from build123d import *

# Parameters (mm, degrees)
F0_W      = 25.4
F0_H      = 25.4
F1_DEPTH  = 25.4
F2_R      = 2.53667
F3_DEPTH  = 5.08
F4_R      = 2.54
F5_DEPTH  = 5.08
F6_R      = 2.54
F7_DEPTH  = 5.08
F8_R      = 2.543532
F9_DEPTH  = 5.08
F10_R     = 2.54
F11_DEPTH = 5.08
F12_R     = 2.54
F13_DEPTH = 5.08
F14_R     = 2.54
F15_DEPTH = 5.08
F16_R     = 2.54
F18_DEPTH = 5.08
F17_R     = 2.54
F19_DEPTH = 5.08
F20_R     = 2.54
F24_DEPTH = 5.08
F23_R     = 2.54
F25_DEPTH = 5.08
F22_R     = 2.54
F26_DEPTH = 5.08
F21_R     = 2.54
F27_DEPTH = 5.08
F28_R     = 2.54
F29_DEPTH = 5.08
F31_R     = 2.54
F32_DEPTH = 5.08
F30_R     = 2.54
F33_DEPTH = 5.08
F34_R     = 2.54
F35_DEPTH = 5.08
F36_R     = 2.54
F37_DEPTH = 5.08
F38_R     = 2.54
F39_DEPTH = 5.08
F40_R     = 2.54
F41_DEPTH = 5.08
F42_R     = 2.54
F43_DEPTH = 5.08


with BuildPart() as f1:
    # F0 (on Top) → F1 (new body)
    with BuildSketch(Plane.XY):
        with Locations((-141.267316, -86.385182)):
            Rectangle(F0_W, F0_H)
    extrude(amount=F1_DEPTH)

    # F2 (on face) → F3 (cut)
    with BuildSketch(Plane(origin=(-153.967316, 0, 0), x_dir=(0, -1, 0), z_dir=(-1, 0, 0))):
        with Locations((86.594619, 12.688329)):
            Circle(F2_R)
    extrude(amount=-F3_DEPTH, mode=Mode.SUBTRACT)

    # F4 (on face) → F5 (cut)
    with BuildSketch(Plane.YZ.offset(-128.567316)):
        with Locations((-91.838241, 17.597279)):
            Circle(F4_R)
    extrude(amount=-F5_DEPTH, mode=Mode.SUBTRACT)

    # F6 (on face) → F7 (cut)
    with BuildSketch(Plane.YZ.offset(-128.567316)):
        with Locations((-79.903536, 17.633894)):
            Circle(F6_R)
    extrude(amount=-F7_DEPTH, mode=Mode.SUBTRACT)

    # F8 (on face) → F9 (cut)
    with BuildSketch(Plane.YZ.offset(-128.567316)):
        with Locations((-79.729639, 10.625202)):
            Circle(F8_R)
    extrude(amount=-F9_DEPTH, mode=Mode.SUBTRACT)

    # F10 (on face) → F11 (cut)
    with BuildSketch(Plane.YZ.offset(-128.567316)):
        with Locations((-91.890648, 11.548187)):
            Circle(F10_R)
    extrude(amount=-F11_DEPTH, mode=Mode.SUBTRACT)

    # F12 (on face) → F13 (cut)
    with BuildSketch(Plane.YZ.offset(-128.567316)):
        with Locations((-92.000924, 5.3013)):
            Circle(F12_R)
    extrude(amount=-F13_DEPTH, mode=Mode.SUBTRACT)

    # F14 (on face) → F15 (cut)
    with BuildSketch(Plane.YZ.offset(-128.567316)):
        with Locations((-79.714611, 4.743482)):
            Circle(F14_R)
    extrude(amount=-F15_DEPTH, mode=Mode.SUBTRACT)

    # F16 (on face) → F18 (cut)
    with BuildSketch(Plane(origin=(0, -73.685182, 0), x_dir=(-1, 0, 0), z_dir=(0, 1, 0))):
        with Locations((141.562238, 9.688065)):
            Circle(F16_R)
    extrude(amount=-F18_DEPTH, mode=Mode.SUBTRACT)

    # F17 (on face) → F19 (cut)
    with BuildSketch(Plane(origin=(0, -73.685182, 0), x_dir=(-1, 0, 0), z_dir=(0, 1, 0))):
        with Locations((151.23339, 17.802121)):
            Circle(F17_R)
    extrude(amount=-F19_DEPTH, mode=Mode.SUBTRACT)

    # F20 (on face) → F24 (cut)
    with BuildSketch(Plane.XY.offset(25.4)):
        with Locations((-139.285192, -92.00193)):
            Circle(F20_R)
    extrude(amount=-F24_DEPTH, mode=Mode.SUBTRACT)

    # F23 (on face) → F25 (cut)
    with BuildSketch(Plane.XY.offset(25.4)):
        with Locations((-150.029391, -92.245251)):
            Circle(F23_R)
    extrude(amount=-F25_DEPTH, mode=Mode.SUBTRACT)

    # F22 (on face) → F26 (cut)
    with BuildSketch(Plane.XY.offset(25.4)):
        with Locations((-138.614863, -80.417737)):
            Circle(F22_R)
    extrude(amount=-F26_DEPTH, mode=Mode.SUBTRACT)

    # F21 (on face) → F27 (cut)
    with BuildSketch(Plane.XY.offset(25.4)):
        with Locations((-148.84156, -82.628928)):
            Circle(F21_R)
    extrude(amount=-F27_DEPTH, mode=Mode.SUBTRACT)

    # F28 (on face) → F29 (cut)
    with BuildSketch(Plane(origin=(0, 0, 0), x_dir=(1, 0, 0), z_dir=(0, 0, -1))):
        with Locations((-137.074172, 86.087316)):
            Circle(F28_R)
    extrude(amount=-F29_DEPTH, mode=Mode.SUBTRACT)

    # F31 (on face) → F32 (cut)
    with BuildSketch(Plane(origin=(0, 0, 0), x_dir=(1, 0, 0), z_dir=(0, 0, -1))):
        with Locations((-151.292577, 86.176708)):
            Circle(F31_R)
    extrude(amount=-F32_DEPTH, mode=Mode.SUBTRACT)

    # F30 (on face) → F33 (cut)
    with BuildSketch(Plane(origin=(0, 0, 0), x_dir=(1, 0, 0), z_dir=(0, 0, -1))):
        with Locations((-144.312844, 86.029641)):
            Circle(F30_R)
    extrude(amount=-F33_DEPTH, mode=Mode.SUBTRACT)

    # F34 (on face) → F35 (cut)
    with BuildSketch(Plane.XZ.offset(99.085182)):
        with Locations((-142.741442, 17.257215)):
            Circle(F34_R)
    extrude(amount=-F35_DEPTH, mode=Mode.SUBTRACT)

    # F36 (on face) → F37 (cut)
    with BuildSketch(Plane.XZ.offset(99.085182)):
        with Locations((-146.107584, 13.017296)):
            Circle(F36_R)
    extrude(amount=-F37_DEPTH, mode=Mode.SUBTRACT)

    # F38 (on face) → F39 (cut)
    with BuildSketch(Plane.XZ.offset(99.085182)):
        with Locations((-141.585246, 9.540573)):
            Circle(F38_R)
    extrude(amount=-F39_DEPTH, mode=Mode.SUBTRACT)

    # F40 (on face) → F41 (cut)
    with BuildSketch(Plane.XZ.offset(99.085182)):
        with Locations((-149.347872, 17.567154)):
            Circle(F40_R)
    extrude(amount=-F41_DEPTH, mode=Mode.SUBTRACT)

    # F42 (on face) → F43 (cut)
    with BuildSketch(Plane.XZ.offset(99.085182)):
        with Locations((-150.112391, 9.50997)):
            Circle(F42_R)
    extrude(amount=-F43_DEPTH, mode=Mode.SUBTRACT)


solid = f1.part
The model under review builds one solid part; all positions refer to its coordinate system, in mm. A direction names the side the tool comes from. Coordinates: 2 decimals unless noted, no trailing zeros. Write each loop counter-clockwise with the first axis right and the second up, starting at its lowest first coordinate (ties: lowest second). Pieces come first, ordered by that corner, then holes. Notation, with made-up numbers: (29, 26.25) - (36, 26.25) arc R8 ccw to (36, 31.25) - close; hole circle Ø8 at (-10, 83.25). An arc over 180 degrees is marked (long way). Answer as CSV lines item,"result".
(1) We need section D-D (x = -138.25). Give the boundary of the cut face in (y, z).
Data:
outline,"(-99.09, 0) - (-88.34, 0) - (-88.34, 5.08) - (-83.84, 5.08) - (-83.84, 0) - (-73.69, 0) - (-73.69, 25.4) - (-77.9, 25.4) - (-77.9, 20.32) - (-82.93, 20.32) - (-82.93, 25.4) - (-89.68, 25.4) - (-89.68, 20.32) - (-94.32, 20.32) - (-94.32, 25.4) - (-99.09, 25.4) - close"
(2) For line 1 along X through (y, z) = (-76.5, 9.5); line 2 along X through (y, z) = (-87, 14); line 3 along Z through (x, y) = (-130.25, -93.5), list the stretches that pass through material, from the lowest coordinate up. Write a range as [from, to].
Data:
line 1,"x = [-153.97, -144.1], [-139.03, -128.57]"
line 2,"x = [-148.89, -128.57]"
line 3,"z = [0, 3.25], [7.35, 9.58], [13.51, 15.68], [19.52, 25.4]"
(3) Tool access review of faces 1 (the cylindrical face through (-131.072, -77.304, 11.389)), 2 (the cylindrical face through (-148.696, -76.19, 17.914)), 3 (the flat face through (-146, -94.005, 13)), 4 (the flat face through (-150, -92, 20.32)), 5 (the cylindrical face through (-138.95, -87.8, 2.5)): name each direction out of +Z, -Z, +X, -X, +Y, -Y from which nothing blocks a thin tool from reaching the whole face with its end or side.
Data:
face 1,"+X"
face 2,"+Y"
face 3,"-Y"
face 4,"+Z"
face 5,"-Z"
(4) Clearance check with flat-ended pins moving along their axes: pin 1 Ø3 at (x, z) = (-146.11, 13.02) entering from -Y; pin 2 Ø8 at (x, y) = (-137.07, -86.09) entering from -Z; pin 3 Ø1 at (y, z) = (-93, 13) entering from +X; pin 4 Ø4.5 at (y, z) = (-86.59, 12.69) entering from -X. State where each tip first meets the part, or that it passes through.
Data:
pin 1,"stops at y = -94.01"
pin 2,"stops at z = 0"
pin 3,"stops at x = -133.65"
pin 4,"stops at x = -148.89"
(5) Mouldability with a two-part tool opening along Z and no side actions: class faces 6 (the flat face through (-153.967, -83.7, 12.5)), 7 (the flat face through (-133.647, -80, 18)), 8 (the flat face through (-139, -80, 20.32)) as pulls with the +Z half, pulls with the -Z half, needs draft (parallel to the pull), parting line crosses it, or undercut.
Data:
face 6,"needs draft"
face 7,"undercut"
face 8,"pulls with the +Z half"
(6) We need section A-A (z = 4). Give the boundary of the cut face in (x, y), plus the area to 3 significant figures.
Data:
outline,"(-153.97, -99.09) - (-128.57, -99.09) - (-128.57, -94.18) - (-133.65, -94.18) - (-133.65, -89.82) - (-128.57, -89.82) - (-128.57, -82.14) - (-133.65, -82.14) - (-133.65, -77.29) - (-128.57, -77.29) - (-128.57, -73.69) - (-153.97, -73.69) - close; hole circle Ø5.08 at (-151.29, -86.18); hole circle Ø5.08 at (-144.31, -86.03); hole circle Ø5.08 at (-137.07, -86.09)"
area,"538 mm2"
(7) We need section B-B (x = -131.5). Give the boundary of the cut face in (y, z), plus the area to 3 significant figures.
Data:
outline,"(-99.09, 0) - (-73.69, 0) - (-73.69, 25.4) - (-99.09, 25.4) - close; hole circle Ø5.08 at (-92, 5.3); hole circle Ø5.08 at (-91.89, 11.55); hole circle Ø5.08 at (-91.84, 17.6); hole circle Ø5.08 at (-79.9, 17.63); hole circle Ø5.09 at (-79.73, 10.63); hole circle Ø5.08 at (-79.71, 4.74)"
area,"523 mm2"
